Source: CAD feature listing. Evaluate the final solid. Frame: model axes, mm. Face numbers are marked on the shaded views. A direction names the side the tool comes from. Give positions to 0.01 mm unless a question says otherwise; leave off trailing zeros. Write each loop counter-clockwise with the first axis right and the second up, starting at its lowest first coordinate (ties: lowest second). Pieces come first, ordered by that corner, then holes. Notation, with made-up numbers: (-17.75, -5.75) - (-0.75, -5.75) arc R26 cw to (-0.75, 20.25) - close; hole circle Ø5 at (61, 76.25). An arc over 180 degrees is marked (long way). One line per question, with ' | ' between items. Start each with the question number.
(1) Pin query (flat end, axial travel): pin 1 (1.1 mm diameter, centred on x = 18.5, z = -3, fed in from -Y); pin 2 (5.5 mm diameter, centred on x = 5.5, y = -2, fed in from -Z); pin 3 (1.1 mm diameter, centred on x = -6.5, z = -2.5, fed in from -Y). Return the tip coordinate at first contact, or that it passes through.
(2) Section A-A, the plane z = -1.25. Return loops of the section in (x, y), plus the area to 3 significant figures.
(3) Ray query, line 1 (Y direction, x = -5.9, z = -1.25); line 2 (X direction, y = -12, z = 2.5); line 3 (X direction, y = -3, z = 2). Return the intervals inside material, ascending. Write a range as [from, to].
(4) Section B-B, the plane y = -9.5. Return loops of the section in (x, z).
(5) Draft query along Y for the marked faces 1, 2, 3 and 4. Return one class per face: +Y half, -Y half, draft (parallel to the pull), parting line (faces both ways), or undercut.
(6) Section C-C, the plane x = 18.5. Return loops of the section in (y, z).
(7) Access query for the marked faces 5, 6 and 7. Directions: +Z, -Z, +X, -X, +Y, -Y. A direction counts if a zero-diameter tool reaches every point of the face in a straight line with its end or side. Return the directions, or none.
(8) Section D-D, the plane y = -1.5. Return loops of the section in (x, z), plus the area to 3 significant figures.
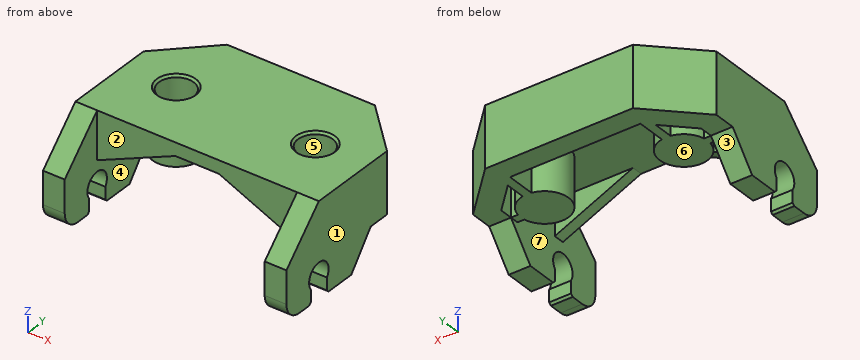
```python
from build123d import *

# Parameters (mm, degrees)
BOSS_EXTRU_1_DEPTH      = 7
CHANFREIN2_SIZE         = 4
CHANFREIN3_SIZE         = 5.5
CHANFREIN4_SIZE         = 5
BOSS_EXTRU_2_DEPTH      = 1.5
ESQUISSE5_W             = 9
ESQUISSE5_H             = 1.25
BOSS_EXTRU_3_DEPTH      = 4
ENL_V_MAT_EXTRU_1_DEPTH = 1.25
ESQUISSE7_R             = 2.75
BOSS_EXTRU_4_DEPTH      = 5.5
ENL_V_START             = -2.5
ESQUISSE9_R             = 2
ENL_V_MAT_EXTRU_2_DEPTH = 4.5
ESQUISSE10_W            = 1.052895571
ESQUISSE10_H            = 1
ESQUISSE10_W_2          = 1
ESQUISSE10_H_2          = 3.75
ESQUISSE10_H_3          = 3.95048694
ESQUISSE10_W_3          = 1.193094599
BOSS_EXTRU_5_DEPTH      = 5.5
ESQUISSE11_W            = 2.5
ESQUISSE11_H            = 10
BOSS_EXTRU_6_DEPTH      = 3.75
ENL_V_MAT_EXTRU_3_DEPTH = 28
ESQUISSE13_W            = 2.5
ESQUISSE13_H            = 3.75
BOSS_EXTRU_7_DEPTH      = 3
ENL_V_MAT_EXTRU_4_DEPTH = 28
CONG_1_R                = 2
CHANFREIN7_SIZE         = 0.25
CHANFREIN8_SIZE         = 0.25


with BuildPart() as part:
    # Esquisse3 → Boss.-Extru.1 (new body)
    with BuildSketch(Plane.XY):
        Polygon((-5.371411117, 0), (17.628588883, 0), (17.628588883, -18.5), (20.128588883, -18.5), (20.128588883, 2.5), (-7.871411117, 2.5), (-7.871411117, -18.5), (-5.371411117, -18.5), align=None)
    extrude(amount=BOSS_EXTRU_1_DEPTH)

    # Chanfrein2
    chanfrein2_edges = [part.edges().sort_by_distance(p)[0] for p in [
        (17.628588883, 0, 3.5),
        (-5.371411117, 0, 3.5),
    ]]
    chamfer(chanfrein2_edges, length=CHANFREIN2_SIZE)

    # Chanfrein3
    chanfrein3_edges = [part.edges().sort_by_distance(p)[0] for p in [
        (-7.871411117, 2.5, 3.5),
        (20.128588883, 2.5, 3.5),
    ]]
    chamfer(chanfrein3_edges, length=CHANFREIN3_SIZE)

    # Chanfrein4
    chanfrein4_edges = [part.edges().sort_by_distance(p)[0] for p in [
        (18.878588883, -18.5, 7),
        (-6.621411117, -18.5, 7),
    ]]
    chamfer(chanfrein4_edges, length=CHANFREIN4_SIZE)

    # Esquisse4 → Boss.-Extru.2 (add)
    with BuildSketch(Plane.XY.offset(7)):
        Polygon((-5.371411117, -13.5), (17.628588883, -13.5), (17.628588883, -4), (13.628588883, 0), (-1.371411117, 0), (-5.371411117, -4), align=None)
    extrude(amount=-BOSS_EXTRU_2_DEPTH)

    # Esquisse5 → Boss.-Extru.3 (add)
    with BuildSketch(Plane(origin=(0, 0, 5.5), x_dir=(-1, 0, 0), z_dir=(0, 0, -1))):
        with Locations((-13.128588883, -12.875)):
            Rectangle(ESQUISSE5_W, ESQUISSE5_H)
        with Locations((0.871411117, -12.875)):
            Rectangle(ESQUISSE5_W, ESQUISSE5_H)
    extrude(amount=BOSS_EXTRU_3_DEPTH)

    # Esquisse6 → Enlèv. mat.-Extru.1 (cut)
    with BuildSketch(Plane.XZ.offset(13.5)):
        Polygon((17.628588883, 1.5), (8.628588883, 5.5), (8.628588883, 1.5), align=None)
        Polygon((-5.371411117, 1.5), (3.628588883, 5.5), (3.628588883, 1.5), align=None)
    extrude(amount=-ENL_V_MAT_EXTRU_1_DEPTH, mode=Mode.SUBTRACT)

    # Esquisse7 → Boss.-Extru.4 (add)
    with BuildSketch(Plane(origin=(0, 0, 5.5), x_dir=(-1, 0, 0), z_dir=(0, 0, -1))):
        with Locations((-14.128588883, -6)):
            Circle(ESQUISSE7_R)
        with Locations((1.871411117, -6)):
            Circle(ESQUISSE7_R)
    extrude(amount=BOSS_EXTRU_4_DEPTH)

    # Esquisse9 → Enlèv. mat.-Extru.2 (cut)
    with BuildSketch(Plane(origin=(0, 0, 0), x_dir=(-1, 0, 0), z_dir=(0, 0, -1)).offset(ENL_V_START)):
        with Locations((-14.128588883, -6)):
            Circle(ESQUISSE9_R)
        with Locations((1.871411117, -6)):
            Circle(ESQUISSE9_R)
    extrude(amount=-ENL_V_MAT_EXTRU_2_DEPTH, mode=Mode.SUBTRACT)

    # Esquisse10 → Boss.-Extru.5 (add)
    with BuildSketch(Plane(origin=(0, 0, 0), x_dir=(-1, 0, 0), z_dir=(0, 0, -1))):
        with Locations((-17.253588884, -6)):
            Rectangle(ESQUISSE10_W, ESQUISSE10_H)
        with Locations((-14.128588883, -1.875)):
            Rectangle(ESQUISSE10_W_2, ESQUISSE10_H_2)
        with Locations((1.871411117, -1.875)):
            Rectangle(ESQUISSE10_W_2, ESQUISSE10_H_3)
        with Locations((4.996411117, -6)):
            Rectangle(ESQUISSE10_W_3, ESQUISSE10_H)
    extrude(amount=-BOSS_EXTRU_5_DEPTH)

    # Esquisse11 → Boss.-Extru.6 (add)
    with BuildSketch(Plane(origin=(0, 0, 0), x_dir=(-1, 0, 0), z_dir=(0, 0, -1))):
        with Locations((6.621411117, -13.5)):
            Rectangle(ESQUISSE11_W, ESQUISSE11_H)
        with Locations((-18.878588883, -13.5)):
            Rectangle(ESQUISSE11_W, ESQUISSE11_H)
    extrude(amount=BOSS_EXTRU_6_DEPTH)

    # Esquisse12 → Enlèv. mat.-Extru.3 (cut)
    with BuildSketch(Plane(origin=(-5.371411117, 0, 0), x_dir=(0, 0, -1), z_dir=(1, 0, 0)).offset(ENL_V_START)):
        with BuildLine():
            Line((3.75, -14.75), (3.75, -12.25))
            Line((3.75, -12.25), (2.079156198, -12.25))
            ThreePointArc((2.079156198, -12.25), (-0.25, -13.5), (2.079156198, -14.75))
            Line((2.079156198, -14.75), (3.75, -14.75))
        make_face()
    extrude(amount=ENL_V_MAT_EXTRU_3_DEPTH, mode=Mode.SUBTRACT)

    # Esquisse13 → Boss.-Extru.7 (add)
    with BuildSketch(Plane(origin=(0, -8.5, 0), x_dir=(1, 0, 0), z_dir=(0, 1, 0))):
        with Locations((18.878588883, 1.875)):
            Rectangle(ESQUISSE13_W, ESQUISSE13_H)
        with Locations((-6.621411117, 1.875)):
            Rectangle(ESQUISSE13_W, ESQUISSE13_H)
    extrude(amount=BOSS_EXTRU_7_DEPTH)

    # Esquisse14 → Enlèv. mat.-Extru.4 (cut)
    with BuildSketch(Plane.ZY.offset(7.871411117)):
        Polygon((-3.75, -5.5), (-3.75, -8.5), (0, -5.5), align=None)
    extrude(amount=-ENL_V_MAT_EXTRU_4_DEPTH, mode=Mode.SUBTRACT)

    # Congé1
    cong_1_edges = [part.edges().sort_by_distance(p)[0] for p in [
        (-6.621411117, -18.5, -3.75),
        (18.878588883, -18.5, -3.75),
    ]]
    fillet(cong_1_edges, radius=CONG_1_R)

    # Chanfrein7
    chanfrein7_edges = [part.edges().sort_by_distance(p)[0] for p in [
        (18.878588883, -14.75, -3.75),
        (18.878588883, -12.25, -3.75),
        (-6.621411117, -12.25, -3.75),
        (-6.621411117, -14.75, -3.75),
    ]]
    chamfer(chanfrein7_edges, length=CHANFREIN7_SIZE)

    # Chanfrein8
    chanfrein8_edges = [part.edges().sort_by_distance(p)[0] for p in [
        (16.128588883, -6, 7),
        (0.128588883, -6, 7),
    ]]
    chamfer(chanfrein8_edges, length=CHANFREIN8_SIZE)


solid = part.part
```
Check sheet entries:
1) pin 1: y = -18.37 | pin 2: z = 0 | pin 3: y = -18.49
2) outline: (-7.87, -18.5) - (-5.37, -18.5) - (-5.37, -15) - (-7.87, -15) - close; (-7.87, -12) - (-5.37, -12) - (-5.37, -6.5) - (-7.87, -6.5) - close; (17.63, -18.5) - (20.13, -18.5) - (20.13, -15) - (17.63, -15) - close; (17.63, -12) - (20.13, -12) - (20.13, -6.5) - (17.63, -6.5) - close | area: 45.0 mm²
3) line 1: [-18.5, -15], [-12, -6.5] | line 2: [-7.87, -5.37], [17.63, 20.13] | line 3: [-7.87, -4.37], [-2.37, -1.37], [13.63, 14.63], [16.63, 20.13]
4) outline: (-7.87, -3.75) - (-5.37, -3.75) - (-5.37, 5.5) - (17.63, 5.5) - (17.63, -3.75) - (20.13, -3.75) - (20.13, 7) - (-7.87, 7) - close
5) face 1: draft | face 2: -Y half | face 3: +Y half | face 4: undercut
6) outline: (-18.5, -1.75) arc R2 ccw to (-16.5, -3.75) - (-15, -3.75) - (-14.75, -3.5) - (-14.75, -2.08) arc R1.5 cw (long way) to (-12.25, -2.08) - (-12.25, -3.5) - (-12, -3.75) - (-8.5, -3.75) - (-5.5, 0) - (-1.37, 0) - (-1.37, 7) - (-13.5, 7) - (-18.5, 2) - close
7) face 5: +Z | face 6: -Z, +Y | face 7: -Z
8) outline: (-6.37, 0) - (-2.87, 0) - (-2.87, 5.5) - (-2.37, 5.5) - (-2.37, 0) - (-1.37, 0) - (-1.37, 5.5) - (13.63, 5.5) - (13.63, 0) - (14.63, 0) - (14.63, 5.5) - (15.13, 5.5) - (15.13, 0) - (18.63, 0) - (18.63, 7) - (-6.37, 7) - close | area: 87.0 mm²
